Can you work these out from the drawing? Everything is in mm from the part's minimum corner. A direction names the side the tool comes from. Round coordinates to 2 decimals unless told otherwise and drop trailing zeros. Write each loop counter-clockwise with the first axis right and the second up, starting at its lowest first coordinate (ties: lowest second). Pieces come first, ordered by that corner, then holes.
Q1. If we section it at A-A (x = 139.7): Please give me the cut outline in (y, z), plus the area to 3 significant figures.
Q2. I'm going to push flat-ended pins straight in: pin 1 Ø9.5 at (x, y) = (133.5, 104) entering from +Z; pin 2 Ø4 at (y, z) = (116.5, 9) entering from +X; pin 3 Ø3 at (y, z) = (15.5, 2) entering from +X; pin 4 Ø6 at (x, y) = (139.7, 12.7) entering from +Z. Where does each tip first touch, or does it pass through?
Q3. Please list where these lines run through material, in increasing order: line 1 along Y through (x, z) = (139.7, 5); line 2 along Y through (x, z) = (135.5, 0.75); line 3 along Y through (x, z) = (124, 2.25).
Q4. If we section it at D-D (y = 99): Please give me the cut outline in (x, z).
Q5. For the marked faces 1, 2, 3, 4 and 5, which set-ups out of +Z, -Z, +X, -X, +Y, -Y let a thin tool reach every point of the face, with its end or its side?
Q6. If we section it at C-C (y = 12.7): Please give me the cut outline in (x, z).
Q7. If we section it at B-B (z = 2.75): Please give me the cut outline in (x, y).
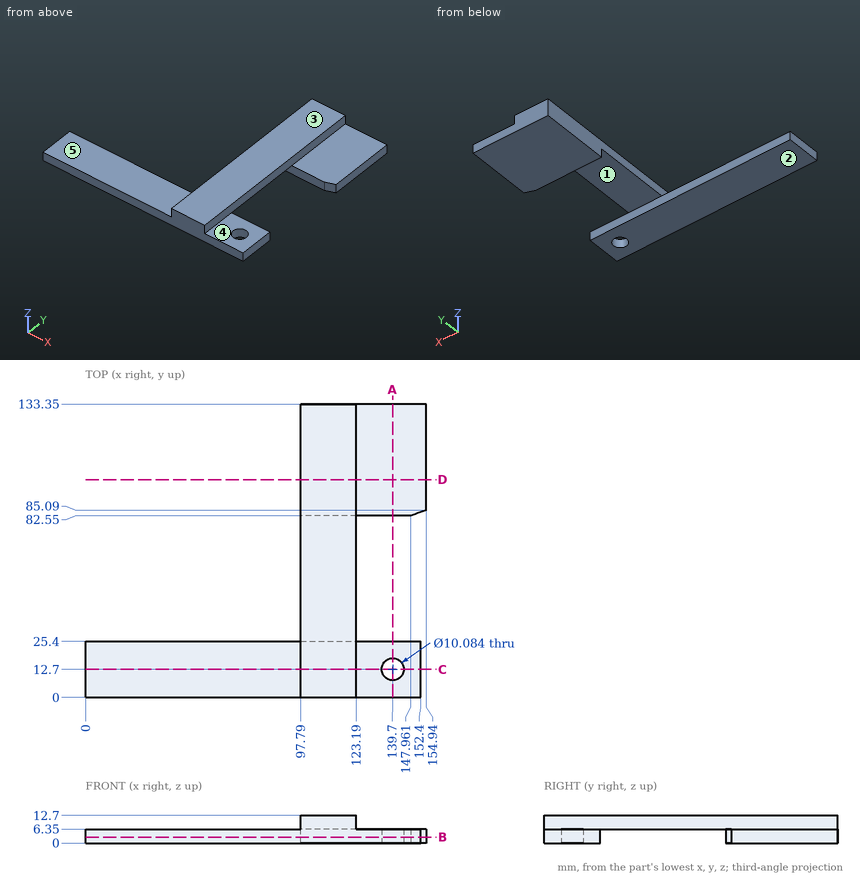
A:
1. outline: (0, 0) - (7.66, 0) - (7.66, 6.35) - (0, 6.35) - close; (17.74, 0) - (25.4, 0) - (25.4, 6.35) - (17.74, 6.35) - close; (82.55, 0) - (133.35, 0) - (133.35, 6.35) - (82.55, 6.35) - close
1. area: 420 mm2
2. pin 1: stops at z = 6.35
2. pin 2: stops at x = 123.19
2. pin 3: stops at x = 152.4
2. pin 4: passes through
3. line 1: y = 0 to 7.66, 17.74 to 25.4, 82.55 to 133.35
3. line 2: y = 0 to 9.91, 15.49 to 25.4, 82.55 to 133.35
3. line 3: y = 0 to 25.4, 82.55 to 133.35
4. outline: (97.79, 0) - (154.94, 0) - (154.94, 6.35) - (123.19, 6.35) - (123.19, 12.7) - (97.79, 12.7) - close
5. face 1: -Z, +X, -X
5. face 2: -Z, +X, -X, +Y, -Y
5. face 3: +Z, +X, -X, +Y, -Y
5. face 4: +Z, +X, +Y, -Y
5. face 5: +Z, -X, +Y, -Y
6. outline: (0, 0) - (134.66, 0) - (134.66, 6.35) - (123.19, 6.35) - (123.19, 12.7) - (97.79, 12.7) - (97.79, 6.35) - (0, 6.35) - close; (144.74, 0) - (152.4, 0) - (152.4, 6.35) - (144.74, 6.35) - close
7. outline: (0, 0) - (152.4, 0) - (152.4, 25.4) - (0, 25.4) - close; (97.79, 82.55) - (147.96, 82.55) - (154.94, 85.09) - (154.94, 133.35) - (97.79, 133.35) - close; hole circle Ø10.08 at (139.7, 12.7)
